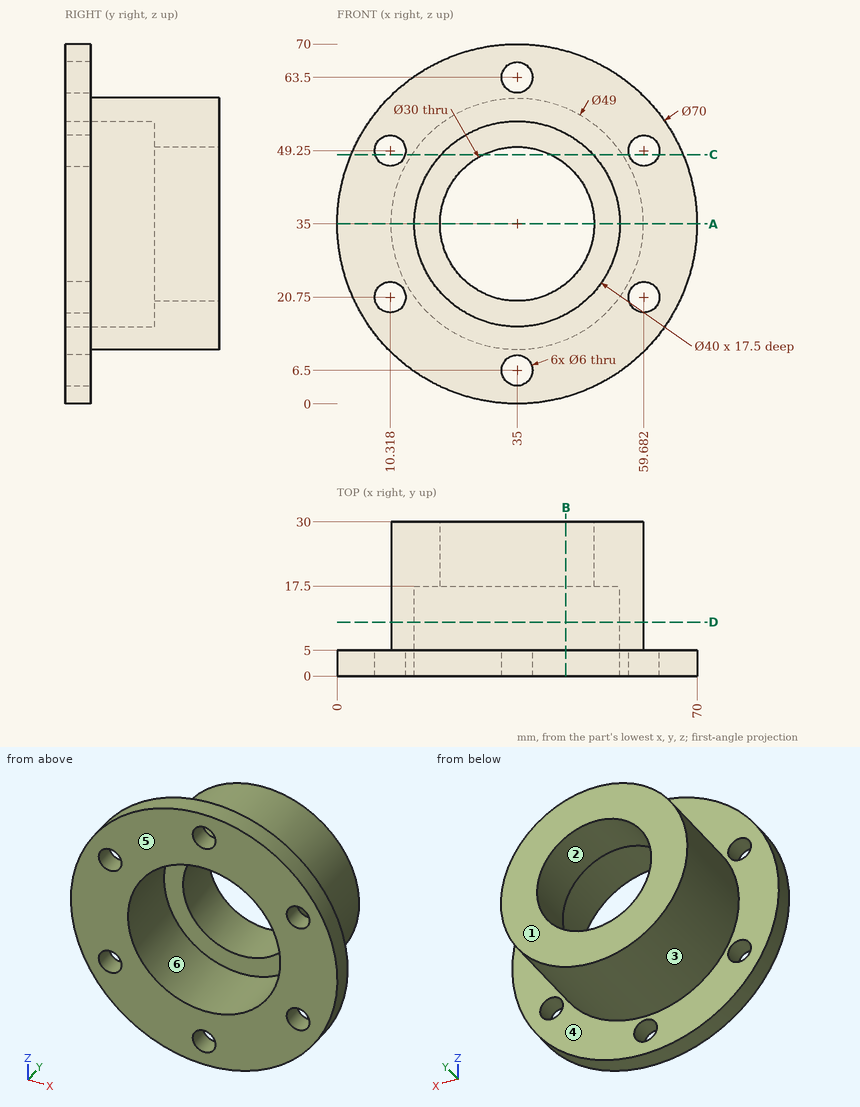
Source: three-view drawing plus pictorial views. Frame: mm from the lowest corner of the part. A direction names the side the tool comes from. Coordinates: 2 decimals unless noted, no trailing zeros. Order: outer loops, then holes, each group sorted by start corner. A loop starts at its lowest first (then second) coordinate and runs counter-clockwise, first axis right, second up.
Item 1: Pull-direction query (X, two-part tool) for the marked faces 1, 2 and 3; classes: pulls with the +X half, pulls with the -X half, needs draft (parallel to the pull), parting line crosses it, or undercut.
Output values:
face 1: needs draft
face 2: undercut
face 3: parting line crosses it
Item 2: Set-up query: the marked faces 4, 5 and 6. Return all of +Z, -Z, +X, -X, +Y, -Y with unobstructed straight access to the full face (end or side cutting, diameter ignored); none if empty.
Output values:
face 4: +Y
face 5: +Z, -Z, +X, -X, -Y
face 6: -Y
Item 3: Cut plane A-A (z = 35). Return loops of the section in (x, y), plus the area to 3 significant figures.
Output values:
outline: (0, 0) - (15, 0) - (15, 17.5) - (20, 17.5) - (20, 30) - (10.5, 30) - (10.5, 5) - (0, 5) - close; (50, 17.5) - (55, 17.5) - (55, 0) - (70, 0) - (70, 5) - (59.5, 5) - (59.5, 30) - (50, 30) - close
area: 500 mm2
Item 4: Material intervals for line 1 (Z direction, x = 35, y = 6); line 2 (X direction, y = 1.5, z = 20.75) (1 decimal); line 3 (Z direction, x = 61, y = 4.25) (1 decimal), sorted ascending.
Output values:
line 1: z = 10.5 to 15, 55 to 59.5
line 2: x = 3 to 7.3, 13.3 to 21, 49 to 56.7, 62.7 to 67
line 3: z = 11.6 to 18.1, 23.4 to 46.6, 51.9 to 58.4
Item 5: Cut plane C-C (z = 48.5). Return loops of the section in (x, y) (1 decimal), plus the area to 3 significant figures.
Output values:
outline: (2.7, 0) - (7.4, 0) - (7.4, 5) - (2.7, 5) - close; (13.2, 0) - (20.2, 0) - (20.2, 17.5) - (28.5, 17.5) - (28.5, 30) - (14.6, 30) - (14.6, 5) - (13.2, 5) - close; (41.5, 17.5) - (49.8, 17.5) - (49.8, 0) - (56.8, 0) - (56.8, 5) - (55.4, 5) - (55.4, 30) - (41.5, 30) - close; (62.6, 0) - (67.3, 0) - (67.3, 5) - (62.6, 5) - close
area: 607 mm2
Item 6: Cut plane D-D (y = 10.5). Return loops of the section in (x, z), plus the area to 3 significant figures.
Output values:
outline: circle Ø49 at (35, 35); hole circle Ø40 at (35, 35)
area: 629 mm2
Item 7: First-contact query: P1, Ø2, axis at y = 21, z = 25, coming from the +X side; P2, Ø1, axis at x = 45, y = 15, coming from the -Z side; P3, Ø1, axis at x = 24.5, y = 9, coming from the -Z side. Flat tips, straight axial feed; report the tip coordinate or a pass-through.
Output values:
P1: stops at x = 57.79
P2: stops at z = 12.42
P3: stops at z = 12.63
Item 8: Cut plane B-B (x = 44.5). Return loops of the section in (y, z).
Output values:
outline: (0, 1.31) - (5, 1.31) - (5, 12.42) - (30, 12.42) - (30, 23.39) - (17.5, 23.39) - (17.5, 17.4) - (0, 17.4) - close; (0, 52.6) - (17.5, 52.6) - (17.5, 46.61) - (30, 46.61) - (30, 57.58) - (5, 57.58) - (5, 68.69) - (0, 68.69) - close
